Verification items for this drawing (mm, ordinates from the low corner). A direction names the side the tool comes from. Give positions to 0.01 mm unless a question says otherwise; leave off trailing zeros. Loops run counter-clockwise (first coordinate to the right, second up) from the corner with the lowest first, then second, coordinate; pieces in that order, holes last. Notation, with made-up numbers: (46.25, 4) -> (60.25, 4) arc R32 ccw to (60.25, 32) -> close; hole circle Ø8 at (-6, 60.5). An arc over 180 degrees is marked (long way). Answer as a JSON object with one key per item and string values.
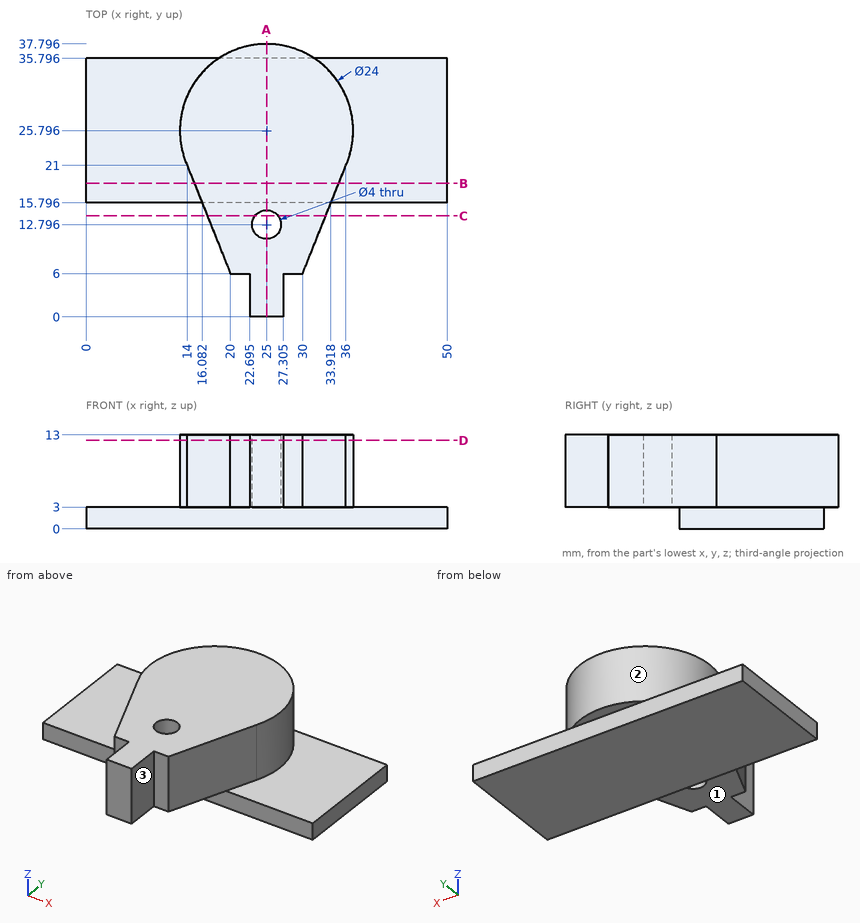
1) Depth check by flat-ended pin: P1, Ø5, axis at x = 21.5, z = 11, coming from the +Y side; P2, Ø12.5, axis at x = 24, y = 5, coming from the -Z side; P3, Ø1.3, axis at x = 29, z = 8.5, coming from the -Y side. Enter the tip coordinate at first touch or a pass-through.
Geometry check:
{"P1": "stops at y = 37.75", "P2": "stops at z = 3", "P3": "stops at y = 6"}
2) Section check B-B on y = 18.5. Record the cut outline in (x, z).
Geometry check:
{"outline": "(0, 0) -> (50, 0) -> (50, 3) -> (35, 3) -> (35, 13) -> (15, 13) -> (15, 3) -> (0, 3) -> close"}
3) Section check D-D on z = 12.25. Record the cut outline in (x, y) (1 decimal).
Geometry check:
{"outline": "(14, 21) -> (20, 6) -> (22.7, 6) -> (22.7, 0) -> (27.3, 0) -> (27.3, 6) -> (30, 6) -> (36, 21) arc R12 ccw (long way) to start; hole circle Ø4 at (25, 12.8)"}
4) Material ranges on line 1 along Y through (x, z) = (25, 7.75); line 2 along X through (y, z) = (13, 5.5); line 3 along Z through (x, y) = (21, 15), recorded low to high. Write a range as from..to.
Geometry check:
{"line 1": "y = 0..10.8, 14.8..37.8", "line 2": "x = 17.2..23.01, 26.99..32.8", "line 3": "z = 3..13"}
5) Section check C-C on y = 14. Record the cut outline in (x, z).
Geometry check:
{"outline": "(16.8, 3) -> (23.4, 3) -> (23.4, 13) -> (16.8, 13) -> close; (26.6, 3) -> (33.2, 3) -> (33.2, 13) -> (26.6, 13) -> close"}
6) Section check A-A on x = 25. Record the cut outline in (y, z).
Geometry check:
{"outline": "(0, 3) -> (10.8, 3) -> (10.8, 13) -> (0, 13) -> close; (14.8, 3) -> (15.8, 3) -> (15.8, 0) -> (35.8, 0) -> (35.8, 3) -> (37.8, 3) -> (37.8, 13) -> (14.8, 13) -> close"}
7) Tool access check on the marked faces 1, 2 and 3. Record the directions out of +Z, -Z, +X, -X, +Y, -Y that give a thin tool (end or side, any length) a straight path to the whole face; none if there is none.
Geometry check:
{"face 1": "-Z, +X, -X, -Y", "face 2": "+Z", "face 3": "+Z, -Z, +X, -Y"}
